Input: part model. Units: mm. Frame: model coordinates. Coordinates: 2 decimals unless noted, no trailing zeros. Write each loop counter-clockwise with the first axis right and the second up, starting at its lowest first coordinate (ties: lowest second). Pieces come first, ordered by that corner, then holes.
1) Section query B-B (x = -12.7). Output: boundary loops of the cut face in (y, z) (1 decimal), then the cut area to 3 significant figures.
2) Section query A-A (z = -0.65). State how many separate pieces and enclosed holes the cut face has, then the cut area to 3 significant figures.
3) Line query: L1, parallel to X at y = -81, z = -2.1; L2, parallel to Y at x = -18, z = -2.7; L3, parallel to Y at x = -33, z = -1.9. Output: solid intervals per line, ascending.
4) Pin query (flat end, axial travel): pin 1 Ø6.5 at (x, y) = (-30.16, -53.53) entering from +Z; pin 2 Ø10 at (x, y) = (-31.43, -1.62) entering from +Z. Return the tip coordinate at first contact, or that it passes through.
from build123d import *

# Parameters (mm, degrees)
BOSS_EXTRUDE1_DEPTH             = 3.175
F_1_2_0_5_DIAMETER_HOLE1_D      = 12.7
F_5_16_0_3125_DIAMETER_HOLE1_D  = 7.9375
F_5_32_0_15625_DIAMETER_HOLE1_D = 3.96875
F_7_64_0_10938_DIAMETER_HOLE1_D = 2.778252
F_6_CLEARANCE_HOLE1_D           = 4.3053
F_16_0_177_DIAMETER_HOLE1_D     = 4.4958


with BuildPart() as part:
    # Sketch1 → Boss-Extrude1 (new body)
    with BuildSketch(Plane.XY):
        with BuildLine():
            Line((-45.72, 26.9875), (-45.72, -84.1375))
            ThreePointArc((-45.72, -84.1375), (-30.833523511, -114.746148224), (-9.525, -141.2875))
            Line((-9.525, -141.2875), (0, -141.2875))
            Line((0, -141.2875), (0, 26.9875))
            Line((0, 26.9875), (-45.72, 26.9875))
        make_face()
    extrude(amount=-BOSS_EXTRUDE1_DEPTH)

    # 1/2 (0.5) Diameter Hole1 (through all)
    with Locations(Plane.XY):
        with Locations((-17.4625, -86.5505), (-31.4325, -1.620345612)):
            Hole(F_1_2_0_5_DIAMETER_HOLE1_D / 2)

    # 5/16 (0.3125) Diameter Hole1 (through all)
    with Locations(Plane.XY):
        with Locations((-22.86, -53.5305)):
            Hole(F_5_16_0_3125_DIAMETER_HOLE1_D / 2)

    # 5/32 (0.15625) Diameter Hole1 (through all)
    with Locations(Plane.XY):
        with Locations((-30.161117219, -53.5305)):
            Hole(F_5_32_0_15625_DIAMETER_HOLE1_D / 2)

    # 7/64 (0.10938) Diameter Hole1 (through all)
    with Locations(Plane.XY):
        with Locations((-17.464635625, -95.966719242), (-31.4325, -11.158858051)):
            Hole(F_7_64_0_10938_DIAMETER_HOLE1_D / 2)

    # #6 Clearance Hole1 (through all)
    with Locations(Plane(origin=(0, 0, -3.175), x_dir=(-1, 0, 0), z_dir=(0, 0, -1))):
        with Locations((12.7, 19.05), (36.3855, -80.4545), (9.144, -122.9995), (31.4325, -24.620045612), (31.4325, 21.404754388)):
            Hole(F_6_CLEARANCE_HOLE1_D / 2)

    # #16 (0.177) Diameter Hole1 (through all)
    with Locations(Plane(origin=(0, 0, -3.175), x_dir=(-1, 0, 0), z_dir=(0, 0, -1))):
        with Locations((12.7, -0.780389216), (12.7, -11.284610784)):
            Hole(F_16_0_177_DIAMETER_HOLE1_D / 2)


solid = part.part
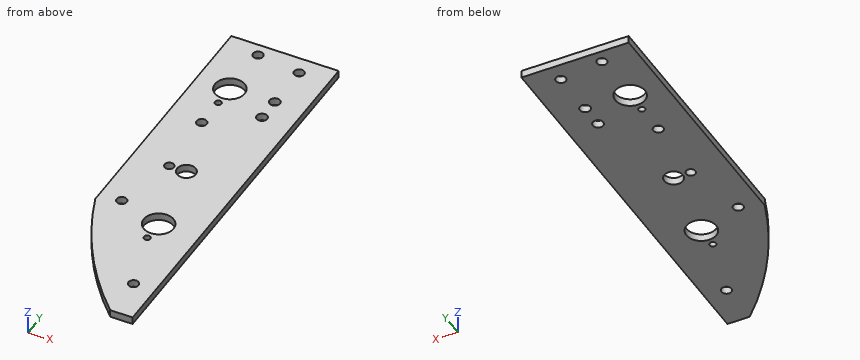
Answer:
1. outline: (-138, -3.2) - (-90.8, -3.2) - (-90.8, 0) - (-138, 0) - close; (-82.4, -3.2) - (-13.5, -3.2) - (-13.5, 0) - (-82.4, 0) - close; (-9, -3.2) - (-3, -3.2) - (-3, 0) - (-9, 0) - close; (1.5, -3.2) - (16.9, -3.2) - (16.9, 0) - (1.5, 0) - close; (21.2, -3.2) - (27, -3.2) - (27, 0) - (21.2, 0) - close
1. area: 455 mm2
2. separate pieces: 1
2. enclosed holes: 13
2. area: 6,400 mm2
3. L1: x = -45.72 to -38.47, -34.3 to -20.55, -14.38 to 0
3. L2: y = -132.14 to -97.25, -94.68 to -92.88, -80.22 to 26.99
3. L3: y = -111.22 to -26.1, -23.14 to -7.77, 4.53 to 19.93, 22.88 to 26.99
4. pin 1: stops at z = 0
4. pin 2: passes through
